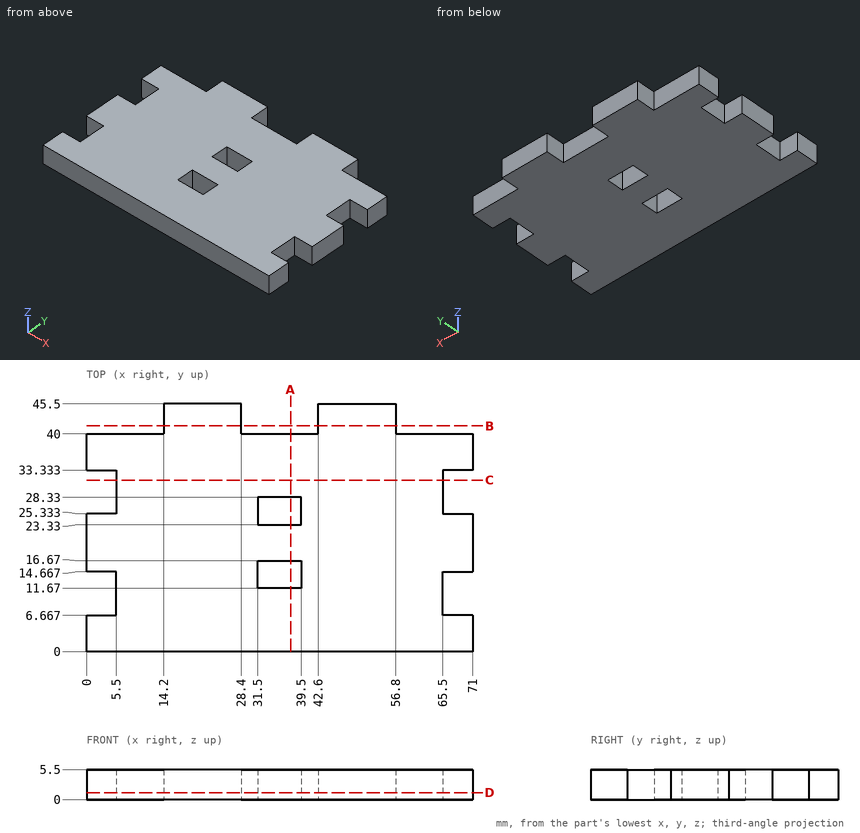
Can you work these out from the drawing? Everything is in mm from the part's minimum corner. Give positions to 0.01 mm unless a question says otherwise; leave off trailing zeros. Write each loop counter-clockwise with the first axis right and the second up, starting at its lowest first coordinate (ties: lowest second). Pieces come first, ordered by that corner, then holes. Notation, with made-up numbers: (-6, 83) -> (16, 83) arc R19 ccw to (16, 108) -> close; hole circle Ø7 at (-33, 85). An arc over 180 degrees is marked (long way). Write each question's results on one line, items separated by ' | '.
Item 1: Suppose I cut it at B-B on y = 41.5. Write out the boundary of the cut face in (x, z).
Output:
outline: (14.2, 0) -> (28.4, 0) -> (28.4, 5.5) -> (14.2, 5.5) -> close; (42.6, 0) -> (56.8, 0) -> (56.8, 5.5) -> (42.6, 5.5) -> close
Item 2: If I drill on L1, parallel to X at y = 15, z = 4.4; L2, parallel to X at y = 43.5, z = 0.4; L3, parallel to Y at x = 8.5, z = 2.45, over which ranges is the centre line in solid material (lowest first)?
Output:
L1: x = 0 to 31.5, 39.5 to 71 | L2: x = 14.2 to 28.4, 42.6 to 56.8 | L3: y = 0 to 40
Item 3: For pin 1 Ø3 at (y, z) = (42, 3.5) entering from -X; pin 2 Ø1 at (x, y) = (16.5, 32) entering from -Z; pin 3 Ø3 at (x, z) = (35, 2) entering from +Y, each with a flat end and sliding along its axis, tell me the tip position at first contact or that it passes through.
Output:
pin 1: stops at x = 14.2 | pin 2: stops at z = 0 | pin 3: stops at y = 40
Item 4: Suppose I cut it at A-A on x = 37.5. Write out the boundary of the cut face in (y, z), plus the area to 3 significant figures.
Output:
outline: (0, 0) -> (11.67, 0) -> (11.67, 5.5) -> (0, 5.5) -> close; (16.67, 0) -> (23.33, 0) -> (23.33, 5.5) -> (16.67, 5.5) -> close; (28.33, 0) -> (40, 0) -> (40, 5.5) -> (28.33, 5.5) -> close | area: 165 mm^2
Item 5: Suppose I cut it at D-D on z = 1.25. Give the number of separate pieces and of enclosed holes in the cut face, plus the area to 3 significant figures.
Output:
separate pieces: 1 | enclosed holes: 2 | area: 2,740 mm^2
Item 6: Suppose I cut it at C-C on y = 31.5. Write out the boundary of the cut face in (x, z), plus the area to 3 significant figures.
Output:
outline: (5.5, 0) -> (65.5, 0) -> (65.5, 5.5) -> (5.5, 5.5) -> close | area: 330 mm^2
